Can you work these out from the drawing? Everything is in mm from the part's minimum corner. Give positions to 0.01 mm unless a question says otherwise; leave off trailing zeros. Loops run counter-clockwise (first coordinate to the right, second up) from the corner with the lowest first, then second, coordinate; pieces in that order, holes last. Notation, with made-up numbers: (-9.5, 5) - (-4.5, 5) arc R14 cw to (-4.5, 11) - close; hole circle Ø6 at (83, 13.25). An arc over 180 degrees is marked (long way). Answer in a Markdown table with one row per item.
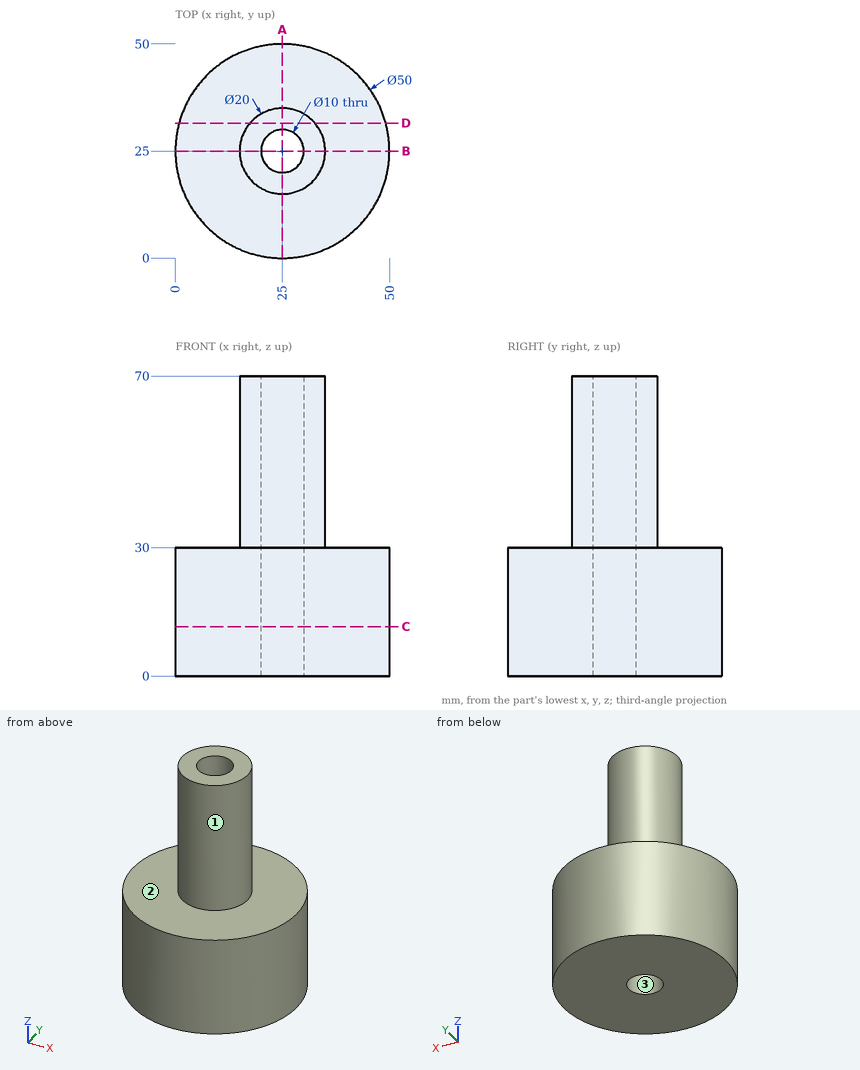
Q1. Imagine slicing it at D-D, the plane y = 31.5. Write out the boundary of the cut face in (x, z).
Checked values:
| item | result |
|---|---|
| outline | (0.86, 0) - (49.14, 0) - (49.14, 30) - (32.6, 30) - (32.6, 70) - (17.4, 70) - (17.4, 30) - (0.86, 30) - close |
Q2. If we mould it in two halves opening along X, with no side actions, what happens to the marked faces 1, 2 and 3? For each: released by +X, released by -X, zero draft, split by the parting line, or undercut.
Checked values:
| item | result |
|---|---|
| face 1 | split by the parting line |
| face 2 | zero draft |
| face 3 | undercut |
Q3. Imagine slicing it at A-A, the plane x = 25. Write out the boundary of the cut face in (y, z), and give its area (3 significant figures).
Checked values:
| item | result |
|---|---|
| outline | (0, 0) - (20, 0) - (20, 70) - (15, 70) - (15, 30) - (0, 30) - close; (30, 0) - (50, 0) - (50, 30) - (35, 30) - (35, 70) - (30, 70) - close |
| area | 1,600 mm² |
Q4. If I drill on line 1 (Y direction, x = 25, z = 41); line 2 (Z direction, x = 30, y = 8); line 3 (X direction, y = 24, z = 18.5), over which ranges is the centre line in solid material (lowest first)? Write a range as [from, to].
Checked values:
| item | result |
|---|---|
| line 1 | y = [15, 20], [30, 35] |
| line 2 | z = [0, 30] |
| line 3 | x = [0.02, 20.1], [29.9, 49.98] |
Q5. Imagine slicing it at C-C, the plane z = 11.5. Write out the boundary of the cut face in (x, y), and give its area (3 significant figures).
Checked values:
| item | result |
|---|---|
| outline | circle Ø50 at (25, 25); hole circle Ø10 at (25, 25) |
| area | 1,880 mm² |
Q6. For pin 1 (1.5 mm diameter, centred on x = 15, z = 24.5, fed in from -Y); pin 2 (1 mm diameter, centred on x = 27, z = 12, fed in from +Y); pin 3 (8 mm diameter, centred on y = 30, z = 8, fed in from +X), each with a flat end and sliding along its axis, tell me the tip position at first contact or that it passes through.
Checked values:
| item | result |
|---|---|
| pin 1 | stops at y = 1.77 |
| pin 2 | stops at y = 49.95 |
| pin 3 | stops at x = 49.98 |
